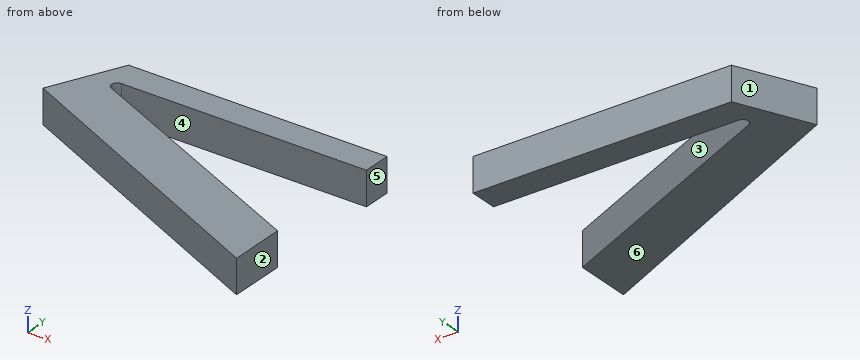
```python
from build123d import *

# Parameters (mm, degrees)
BOSS_EXTRUDE1_DEPTH      = 3
BOSS_EXTRUDE1_DEPTH_BACK = 3
FILLET1_R                = 1


with BuildPart() as part:
    # Sketch2 → Boss-Extrude1 (new, two sides: drawn at the far end of the back side and taken through both)
    with BuildSketch(Plane.XY.offset(-BOSS_EXTRUDE1_DEPTH_BACK)):
        Polygon((0, 0), (0, -5), (-48.01, -5), (0.217510674, -26.897270955), (0.217510674, -36.897270955), (-51.661084359, -12.686242943), (-45.74, 0), align=None)
    extrude(amount=BOSS_EXTRUDE1_DEPTH + BOSS_EXTRUDE1_DEPTH_BACK)

    # Fillet1
    fillet1_edges = [part.edges().sort_by_distance(p)[0] for p in [
        (-48.01, -5, 0),
    ]]
    fillet(fillet1_edges, radius=FILLET1_R)


solid = part.part
```
For this review, take the finished solid that the model builds, in its own axes (mm). Face numbers are marked on the shaded views. A direction names the side the tool comes from. Round coordinates to 2 decimals unless told otherwise and drop trailing zeros. Write each loop counter-clockwise with the first axis right and the second up, starting at its lowest first coordinate (ties: lowest second). Pieces come first, ordered by that corner, then holes. Notation, with made-up numbers: (-29.75, -16) - (3.25, -16) arc R27 cw to (3.25, 9) - close; hole circle Ø7 at (42.5, 86). An arc over 180 degrees is marked (long way). Use CSV: the item, a comma, the result in double quotes.
1) Clearance check with flat-ended pins moving along their axes: pin 1 Ø3 at (x, z) = (-33.5, -2) entering from -Y; pin 2 Ø3 at (x, z) = (-28, -1) entering from +Y; pin 3 Ø2 at (y, z) = (-8, -1.5) entering from -X; pin 4 Ø1.8 at (x, z) = (-29, 0.5) entering from -Y. State where each tip first meets the part, or that it passes through.
Conclusion:
pin 1,"stops at y = -21.86"
pin 2,"stops at y = 0"
pin 3,"stops at x = -49.94"
pin 4,"stops at y = -23.68"
2) Wall thickness on line 1 along Y through (x, z) = (-29, -2.4); line 2 along Y through (x, z) = (-12, -0.2); line 3 along Y through (x, z) = (-47.5, -0.65): over which ranges is each line inside the solid? List them lowest first. Write a range as from..to.
Conclusion:
line 1,"y = -23.26..-13.63, -5..0"
line 2,"y = -31.2..-21.35, -5..0"
line 3,"y = -14.63..-3.77"
3) Add section D-D on y = -32.5. Write out the cut boundary in (x, z), and give its area (3 significant figures).
Conclusion:
outline,"(-9.2, -3) - (0.22, -3) - (0.22, 3) - (-9.2, 3) - close"
area,"56.5 mm^2"
4) The part is to be moulded in two halves that separate along Y. For the marked faces 1, 2 and 3, say which applies: pulls with the +Y half, pulls with the -Y half, needs draft (parallel to the pull), parting line crosses it, or undercut.
Conclusion:
face 1,"pulls with the +Y half"
face 2,"needs draft"
face 3,"undercut"
5) For the marked faces 4, 5 and 6, list the 3-axis set-ups (+Z, -Z, +X, -X, +Y, -Y) from which the entire face can be reached by the end or side of a thin tool; tool diameter is ignored.
Conclusion:
face 4,"+Z, -Z, +X"
face 5,"+Z, -Z, +X, +Y"
face 6,"-Z, +X, -X, +Y, -Y"
6) Add section C-C on x = -14. Write out the cut boundary in (y, z).
Conclusion:
outline,"(-30.26, -3) - (-20.44, -3) - (-20.44, 3) - (-30.26, 3) - close; (-5, -3) - (0, -3) - (0, 3) - (-5, 3) - close"
7) Add section A-A on x = -42. Write out the cut boundary in (y, z).
Conclusion:
outline,"(-17.19, -3) - (-7.73, -3) - (-7.73, 3) - (-17.19, 3) - close; (-5, -3) - (0, -3) - (0, 3) - (-5, 3) - close"
8) Add section B-B on z = 1.45. Write out the cut boundary in (x, y).
Conclusion:
outline,"(-51.66, -12.69) - (0.22, -36.9) - (0.22, -26.9) - (-43.8, -6.91) arc R1 cw to (-43.39, -5) - (0, -5) - (0, 0) - (-45.74, 0) - close"
